Check sheet for the modelled part. Datum: model origin and axes. Units: mm. A direction names the side the tool comes from. Coordinates: 2 decimals unless noted, no trailing zeros. Answer as CSV lines item,"result". Start each with the question number.
from build123d import *

# Parameters (mm, degrees)
F1_DEPTH = 19.05
F3_D     = 25.4
F3_DEPTH = 63.5
F3_TIP   = 7.6309298617
F5_DEPTH = 50.4981949925
F7_DEPTH = 40.6211540103
F9_D     = 6.35
F11_D    = 6.35


with BuildPart() as f1:
    # F0 (on Right) → F1 (new body, symmetric)
    with BuildSketch(Plane.YZ):
        Polygon((242.8656616081, 21.4498834579), (-61.9343383919, -29.3501165421), (-61.9343383919, -54.7501165421), (242.8656616081, -54.7501165421), align=None)
    extrude(amount=F1_DEPTH, both=True)

    # F3
    with Locations(Plane(origin=(0, 242.8656616081, 0), x_dir=(-1, 0, 0), z_dir=(0, 1, 0))):
        with Locations((-0.3272963222, -16.9025734067)):
            Hole(F3_D / 2, depth=F3_DEPTH)
            with Locations((0, 0, -(F3_DEPTH + F3_TIP / 2))):  # 118° drill point
                Cone(0, F3_D / 2, F3_TIP, mode=Mode.SUBTRACT)

    # F4 (on face) → F5 (cut)
    with BuildSketch(Plane(origin=(-19.05, 0, 0), x_dir=(0, -1, 0), z_dir=(-1, 0, 0))):
        with BuildLine():
            Line((61.9343383919, -29.3501165421), (-217.434808525, 17.2114079441))
            add(Edge.make_bspline(
                [(-217.434808525, 17.2114079441), (-181.7031574212, 2.796838546), (-103.7756395376, -28.6400418614), (3.7252200382, -29.1006886434), (61.9343383919, -29.3501165421)],
                knots=[0, 0, 0, 0, 0.4585241666, 1, 1, 1, 1], degree=3))
        make_face()
    extrude(amount=-F5_DEPTH, mode=Mode.SUBTRACT)

    # F6 (on face) → F7 (cut)
    with BuildSketch(Plane(origin=(-19.05, 0, 0), x_dir=(0, -1, 0), z_dir=(-1, 0, 0))):
        with BuildLine():
            add(Edge.make_bspline(
                [(61.9343383919, -51.728207618), (53.7275699574, -49.4475771186), (38.4988179682, -45.1515261487), (31.8427817105, -34.270455265), (28.7836416426, -29.1453393273)],
                knots=[0, 0, 0, 0, 0.5369777676, 1, 1, 1, 1], degree=3))
            Line((61.9343383919, -51.728207618), (61.9343383919, -29.3501165421))
            add(Edge.make_bspline(
                [(28.7836416426, -29.1453393273), (39.7941135042, -29.2552449401), (50.8642259332, -29.3026807628), (61.9343383919, -29.3501165421)],
                knots=[0.8970230345, 0.8970230345, 0.8970230345, 0.8970230345, 1, 1, 1, 1], degree=3))
        make_face()
    extrude(amount=-F7_DEPTH, mode=Mode.SUBTRACT)

    # F9 (through all)
    with Locations(Plane(origin=(-19.05, 0, 0), x_dir=(0, -1, 0), z_dir=(-1, 0, 0))):
        with Locations((30.7875052094, -48.9864274859)):
            Hole(F9_D / 2)

    # F11 (through all)
    with Locations(Plane(origin=(-19.05, 0, 0), x_dir=(0, -1, 0), z_dir=(-1, 0, 0))):
        with Locations((-229.6800166368, -39.5821034908)):
            Hole(F11_D / 2)


solid = f1.part
Item 1: Set-up check for faces 1 (the face through (-1.33, 210.67, -4.31)), 2 (the face through (0.27, 226.51, -39.44)): record each of +Z, -Z, +X, -X, +Y, -Y from which the full face is reachable in a straight line by a thin tool's end or side.
Item 2: Release check for a two-part mould opening along X. For faces 3 (the face through (-0.69, 173.06, -18.86)), 4 (the face through (0, 88, -54.75)), 5 (the face through (19.05, 122, -33)) record: released by +X, released by -X, zero draft, split by the parting line, or undercut.
Item 3: Go/stop test with flat-tipped pins: pin 1 (8 mm diameter, centred on x = -7, y = 153.5, fed in from +Z); pin 2 (5 mm diameter, centred on x = -11, z = -30, fed in from -Y). Record where each tip stops, or that it passes through.
Item 4: Sectioned sample at A-A, the plane x = -8. Give the number of separate pieces and of enclosed holes in the cut face, and give its area (3 significant figures).
Item 5: Material ranges on line 1 (Z direction, x = -11, y = -24.5); line 2 (X direction, y = 203, z = -8.5); line 3 (Y direction, x = -11.5, z = -37), recorded low to high. Write a range as from..to.
Reply:
1,face 1,"+Y"
1,face 2,"+X, -X"
2,face 3,"undercut"
2,face 4,"zero draft"
2,face 5,"released by +X"
3,pin 1,"z = -5.47"
3,pin 2,"y = -30.82"
4,separate pieces,"1"
4,enclosed holes,"2"
4,area,"10,500 mm²"
5,line 1,"-54.75..-29.1"
5,line 2,"-19.05..-9.2, 9.85..19.05"
5,line 3,"-33.92..227.83, 231.53..242.87"
